```python
from build123d import *

# Parameters (mm, degrees)
ESQUISSE1_W                     = 100
ESQUISSE1_H                     = 85
BOSS_EXTRU_1_DEPTH              = 5
ESQUISSE2_R                     = 1.5
ENL_V_MAT_EXTRU_1_DEPTH         = 85
ESQUISSE3_R                     = 1.375
ENL_V_MAT_EXTRU_2_DEPTH         = 5
R_P_TITION_LIN_AIRE1_COUNT      = 7
R_P_TITION_LIN_AIRE1_PITCH      = 11.5
R_P_TITION_LIN_AIRE1_COUNT_DIR2 = 6
R_P_TITION_LIN_AIRE1_PITCH_DIR2 = 14.5
ESQUISSE4_R                     = 1.5
ENL_V_MAT_EXTRU_3_DEPTH         = 5
CONG_1_R                        = 1


with BuildPart() as part:
    # Esquisse1 → Boss.-Extru.1 (new body)
    with BuildSketch(Plane(origin=(0, 0, 0), x_dir=(1, 0, 0), z_dir=(0, 1, 0))):
        Rectangle(ESQUISSE1_W, ESQUISSE1_H)
    extrude(amount=BOSS_EXTRU_1_DEPTH)

    # Esquisse2 → Enlèv. mat.-Extru.1 (cut)
    with BuildSketch(Plane.XY.offset(42.5)):
        with Locations((-25, 2.5)):
            Circle(ESQUISSE2_R)
        with Locations((25, 2.5)):
            Circle(ESQUISSE2_R)
    extrude(amount=-ENL_V_MAT_EXTRU_1_DEPTH, mode=Mode.SUBTRACT)

    # Esquisse3 → Enlèv. mat.-Extru.2 (cut)
    with BuildSketch(Plane(origin=(0, 0, 0), x_dir=(1, 0, 0), z_dir=(0, 1, 0))):
        with Locations(Location((-36.5, 34.5, 0), (0, 0, 90))):
            Circle(ESQUISSE3_R)
    enl_v_mat_extru_2 = extrude(amount=ENL_V_MAT_EXTRU_2_DEPTH, mode=Mode.SUBTRACT)

    # Répétition linéaire1: Enl_v. mat.-Extru.2 7 × 6
    with Locations(*[(j * R_P_TITION_LIN_AIRE1_PITCH_DIR2, 0, i * R_P_TITION_LIN_AIRE1_PITCH) for i in range(R_P_TITION_LIN_AIRE1_COUNT) for j in range(R_P_TITION_LIN_AIRE1_COUNT_DIR2) if (i, j) != (0, 0)]):
        add(enl_v_mat_extru_2, mode=Mode.SUBTRACT)

    # Esquisse4 → Enlèv. mat.-Extru.3 (cut)
    with BuildSketch(Plane(origin=(0, 0, 0), x_dir=(1, 0, 0), z_dir=(0, 1, 0))):
        with Locations(Location((-47.5, 0, 0), (0, 0, 90))):
            Circle(ESQUISSE4_R)
        with Locations(Location((47.5, 0, 0), (0, 0, 90))):
            Circle(ESQUISSE4_R)
    extrude(amount=ENL_V_MAT_EXTRU_3_DEPTH, mode=Mode.SUBTRACT)

    # Congé1
    cong_1_edges = [part.edges().sort_by_distance(p)[0] for p in [
        (-50, 0, 0),
        (50, 0, 0),
    ]]
    fillet(cong_1_edges, radius=CONG_1_R - 0.0001)  # a hair under: the kernel refuses the full size


solid = part.part
```
Can you work these out from the model? Positions are in its coordinate system, mm. Round coordinates to 2 decimals unless told otherwise and drop trailing zeros. Loops run counter-clockwise (first coordinate to the right, second up) from the corner with the lowest first, then second, coordinate; pieces in that order, holes last. Notation, with made-up numbers: (32.25, -34) -> (80.25, -34) arc R34 ccw to (80.25, -4) -> close; hole circle Ø2 at (16.25, -37). An arc over 180 degrees is marked (long way). Answer in a Markdown table with one row per item.
Item 1: We'd pull the mould along Z, two halves only. Please class faces 1 (the flat face through (-1, 2, 42.5)), 2 (the cylindrical face through (35.071, 2.465, -21.987)), 3 (the flat face through (-1, 0, -1)), 4 (the cylindrical face through (-7.56, 2.465, 12.874)): released by +Z, released by -Z, zero draft, split by the parting line, or undercut.
Answer block:
| item | result |
|---|---|
| face 1 | released by +Z |
| face 2 | undercut |
| face 3 | zero draft |
| face 4 | undercut |
Item 2: Suppose I cut it at C-C, the plane z = 5.5. List the corners of the cut face in (x, y) for me.
Answer block:
| item | result |
|---|---|
| outline | (-50, 1) arc R1 ccw to (-49, 0) -> (49, 0) arc R1 ccw to (50, 1) -> (50, 5) -> (-50, 5) -> close; hole circle Ø3 at (-25, 2.5); hole circle Ø3 at (25, 2.5) |
Item 3: Suppose I cut it at A-A, the plane z = 34.5. Give the number of separate pieces and of enclosed holes in the cut face, plus the area to 3 significant figures.
Answer block:
| item | result |
|---|---|
| separate pieces | 7 |
| enclosed holes | 2 |
| area | 403 mm² |
Item 4: Suppose I cut it at B-B, the plane x = -47.5. List the corners of the cut face in (y, z) for me, plus the area to 3 significant figures.
Answer block:
| item | result |
|---|---|
| outline | (0, -42.5) -> (5, -42.5) -> (5, -1.5) -> (0, -1.5) -> close; (0, 1.5) -> (5, 1.5) -> (5, 42.5) -> (0, 42.5) -> close |
| area | 410 mm² |
Item 5: If I drill on probe 1 along X at (y, z) = (2.55, -8); probe 2 along Y at (x, z) = (24, 18); probe 3 along X at (y, z) = (0.45, -21), over which ranges is the centre line in solid material (lowest first)?
Answer block:
| item | result |
|---|---|
| probe 1 | -50 to -26.5, -23.5 to 23.5, 26.5 to 50 |
| probe 2 | 0 to 1.38, 3.62 to 5 |
| probe 3 | -49.84 to 49.84 |
